```python
from build123d import *

# Parameters (mm, degrees)
F0_W     = 50
F0_H     = 50
F1_DEPTH = 50
F3_DEPTH = 50
F5_DEPTH = 50
F7_DEPTH = 50


with BuildPart() as f1:
    # F0 (on Top) → F1 (new body)
    with BuildSketch(Plane.XY):
        Rectangle(F0_W, F0_H)
    extrude(amount=F1_DEPTH)

    # F2 (on face) → F3 (cut)
    with BuildSketch(Plane(origin=(-25, 0, 0), x_dir=(0, -1, 0), z_dir=(-1, 0, 0))):
        Polygon((17, 24.999999), (0, 42), (-17, 25.000001), (0, 8), align=None)
    extrude(amount=-F3_DEPTH, mode=Mode.SUBTRACT)

    # F4 (on face) → F5 (cut)
    with BuildSketch(Plane.XZ.offset(25)):
        Polygon((17, 24.999998), (0, 42), (-17, 25.000002), (0, 8), align=None)
    extrude(amount=-F5_DEPTH, mode=Mode.SUBTRACT)

    # F6 (on face) → F7 (cut)
    with BuildSketch(Plane.XY.offset(50)):
        Polygon((17, 0), (0, 17), (-17, 0), (0, -17), align=None)
    extrude(amount=-F7_DEPTH, mode=Mode.SUBTRACT)


solid = f1.part
```
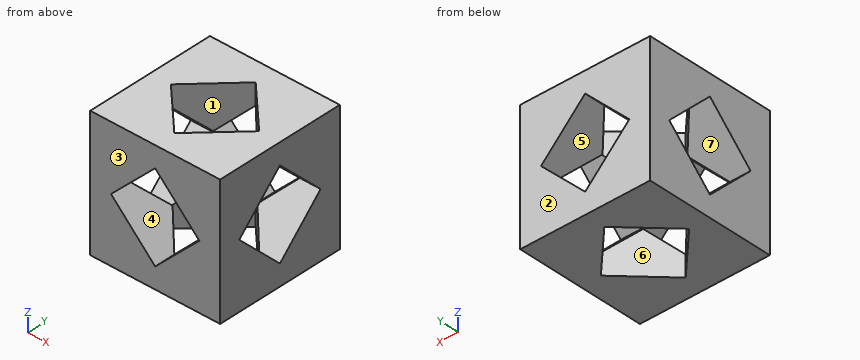
Design review of the part built by this model. Coordinates are the model's own, in mm. Face numbers are marked on the shaded views. A direction names the side the tool comes from. Give positions to 0.01 mm unless a question says otherwise; leave off trailing zeros. Loops run counter-clockwise (first coordinate to the right, second up) from the corner with the lowest first, then second, coordinate; pieces in that order, holes last. Notation, with made-up numbers: M 50.5,-19.75 L 96.5,-19.75 A35 ccw 96.5,12.25 Z; hole C 5.5,56.25 d4. An arc over 180 degrees is marked long. Return JSON: item names as keys, results as strings. Group by question number.
Item 1: We need section D-D (x = -19). Give the boundary of the cut face in (y, z), and give its area (3 significant figures).
Item 2: Mouldability with a two-part tool opening along Y and no side actions: class the marked faces 1, 2, 3 and 4 as released by +Y, released by -Y, zero draft, split by the parting line, or undercut.
Item 3: Insertion check: pin 1 Ø10 at (x, y) = (2, 4.5) entering from -Z. The pin has a flat end and moves straight along its axis. Give the tip position at first contact, or say it passes through.
Item 4: We need section C-C (x = -13). Give the boundary of the cut face in (y, z).
Item 5: For probe 1 along Y at (x, z) = (0, 47.5); probe 2 along X at (y, z) = (19.5, 38); probe 3 along X at (y, z) = (17.5, 34.5), list the stretches that pass through material, from the lowest coordinate up.
Item 6: We need section A-A (z = 11). Give the boundary of the cut face in (x, y).
Item 7: Tool access review of the marked faces 5, 6 and 7: name each direction out of +Z, -Z, +X, -X, +Y, -Y from which nothing blocks a thin tool from reaching the whole face with its end or side.
Item 8: We need section B-B (y = -3.5). Give the boundary of the cut face in (x, z), and give its area (3 significant figures).
Output:
{
 "1": {"outline": "M -25,0 L 25,0 L 25,50 L -25,50 Z; hole M -17,25 L 0,8 L 17,25 L 0,42 Z", "area": "1,920 mm^2"},
 "2": {"face 1": "undercut", "face 2": "released by +Y", "face 3": "released by -Y", "face 4": "zero draft"},
 "3": {"pin 1": "passes through"},
 "4": {"outline": "M -25,0 L -4,0 L -4,12 L -13,21 L -25,21 Z; M -25,29 L -13,29 L -4,38 L -4,50 L -25,50 Z; M 4,0 L 25,0 L 25,21 L 13,21 L 4,12 Z; M 4,38 L 13,29 L 25,29 L 25,50 L 4,50 Z"},
 "5": {"probe 1": "y = -25 to -17, 17 to 25", "probe 2": "x = -25 to -4, 4 to 25", "probe 3": "x = -25 to -7.5, 7.5 to 25"},
 "6": {"outline": "M -25,-25 L -3,-25 L -3,-14 L -14,-3 L -25,-3 Z; M -25,3 L -14,3 L -3,14 L -3,25 L -25,25 Z; M 3,-25 L 25,-25 L 25,-3 L 14,-3 L 3,-14 Z; M 3,14 L 14,3 L 25,3 L 25,25 L 3,25 Z"},
 "7": {"face 5": "+Y, -Y", "face 6": "+Z, -Z", "face 7": "+X, -X"},
 "8": {"outline": "M -25,0 L -13.5,0 L -13.5,11.5 L -25,11.5 Z; M -25,38.5 L -13.5,38.5 L -13.5,50 L -25,50 Z; M 13.5,0 L 25,0 L 25,11.5 L 13.5,11.5 Z; M 13.5,38.5 L 25,38.5 L 25,50 L 13.5,50 Z", "area": "529 mm^2"}
}
